For this review, take the finished solid that the model builds, in its own axes (mm). A direction names the side the tool comes from. Round coordinates to 2 decimals unless told otherwise and drop trailing zeros. Order: outer loops, then holes, each group sorted by start corner. A loop starts at its lowest first (then second) coordinate and runs counter-clockwise, first axis right, second up.
```python
from build123d import *

# Parameters (mm, degrees)
ESQUISSE1_W             = 50
ESQUISSE1_H             = 25
BOSS_EXTRU_1_DEPTH      = 12.5
ESQUISSE2_R             = 5
BOSS_EXTRU_2_DEPTH      = 10
BOSS_EXTRU_2_TAPER      = 10
ESQUISSE4_R             = 5
BOSS_EXTRU_3_DEPTH      = 10
BOSS_EXTRU_3_TAPER      = 10
ENL_V_MAT_EXTRU_5_DEPTH = 26
ESQUISSE14_R            = 1.5
ENL_V_MAT_EXTRU_6_DEPTH = 4
ENL_V_MAT_EXTRU_6_TAPER = 10


with BuildPart() as part:
    # Esquisse1 → Boss.-Extru.1 (new body)
    with BuildSketch(Plane(origin=(0, 0, 0), x_dir=(1, 0, 0), z_dir=(0, 1, 0))):
        Rectangle(ESQUISSE1_W, ESQUISSE1_H)
    extrude(amount=-BOSS_EXTRU_1_DEPTH)

    # Esquisse2 → Boss.-Extru.2 (add)
    with BuildSketch(Plane.XZ.offset(12.5)):
        with Locations((17, 4.5)):
            Circle(ESQUISSE2_R)
    extrude(amount=BOSS_EXTRU_2_DEPTH, taper=BOSS_EXTRU_2_TAPER)

    # Esquisse4 → Boss.-Extru.3 (add)
    with BuildSketch(Plane.XZ.offset(12.5)):
        with Locations((-17, -4.5)):
            Circle(ESQUISSE4_R)
    extrude(amount=BOSS_EXTRU_3_DEPTH, taper=BOSS_EXTRU_3_TAPER)

    # Esquisse6 → Enlèvement de matière-Révolution1 (revolve, cut)
    with BuildSketch(Plane.XY):
        with BuildLine():
            Line((0, -20), (0, -5))
            ThreePointArc((0, -5), (-7.5, -12.5), (0, -20))
        make_face()
    revolve(axis=Axis((0, -20, 0), (0, 1, 0)), mode=Mode.SUBTRACT)

    # Esquisse8 → Enlèvement de matière-Révolution2 (revolve, cut)
    with BuildSketch(Plane.XY):
        with BuildLine():
            Line((8, -12.5), (10, -12.5))
            ThreePointArc((10, -12.5), (9, -11.5), (8, -12.5))
        make_face()
    revolve(axis=Axis((0, -20, 0), (0, 1, 0)), mode=Mode.SUBTRACT)

    # Esquisse13 → Enlèv. mat.-Extru.5 (cut, through all)
    with BuildSketch(Plane(origin=(0, 0, -12.5), x_dir=(-1, 0, 0), z_dir=(0, 0, -1))):
        Polygon((20, 0), (20, -7.5), (10, -7.5), (10, -2.5), (-10, -2.5), (-10, -7.5), (-20, -7.5), (-20, 0), align=None)
    extrude(amount=-ENL_V_MAT_EXTRU_5_DEPTH, mode=Mode.SUBTRACT)

    # Esquisse14 → Enlèv. mat.-Extru.6 (cut)
    with BuildSketch(Plane.XY.offset(12.5)):
        with Locations((0, -12.5)):
            Circle(ESQUISSE14_R)
    extrude(amount=-ENL_V_MAT_EXTRU_6_DEPTH, taper=ENL_V_MAT_EXTRU_6_TAPER, mode=Mode.SUBTRACT)


solid = part.part
```
Q1. Take a section at B-B, the plane y = -10.25. State the section outline as (x, z) points, plus the area to 3 significant figures.
Q2. Clearance check with a flat-ended pin moving along its axis: pin 1 (6 mm diameter, centred on x = -2.5, z = 3.5, fed in from +Y). State where the tip first meets the part, or that it passes through.
Q3. Tool access review of faces 1 (the face through (5, -12.5, 6)), 2 (the face through (0, -2.5, 0)), 3 (the face through (-6, -12.5, -9)), 4 (the face through (22, 0, 0)): name each direction out of +Z, -Z, +X, -X, +Y, -Y from which nothing blocks a thin tool from reaching the whole face with its end or side.
Q4. Wall thickness on line 1 (X direction, y = -3.5, z = -5); line 2 (X direction, y = -1.5, z = 0.5); line 3 (Y direction, x = -18.5, z = -10.25): over which ranges is each line inside the solid? List them lowest first.
Q5. Take a section at C-C, the plane x = 0. State the section outline as (y, z) points, plus the area to 3 significant figures.
Q6. Take a section at A-A, the plane x = -17. State the section outline as (y, z) points.
Working result:
1. outline: (-25, -12.5) - (25, -12.5) - (25, 12.5) - (-25, 12.5) - close; hole circle Ø14.31 at (0, 0)
1. area: 1,090 mm2
2. pin 1: stops at y = -2.5
3. face 1: +Z, -Z, -Y
3. face 2: +Z, -Z, +Y
3. face 3: -Y
3. face 4: +Z, -Z, +X, -X, +Y
4. line 1: x = -25 to -20, -10 to 10, 20 to 25
4. line 2: x = -25 to -20, 20 to 25
4. line 3: y = -12.5 to -7.5
5. outline: (-12.5, -12.5) - (-2.5, -12.5) - (-2.5, 12.5) - (-11, 12.5) - (-11.56, 9.34) arc R1 cw to (-12.5, 8) - (-12.5, 7.5) arc R7.5 cw to (-12.5, -7.5) - (-12.5, -8) arc R1 cw to (-12.5, -10) - close
5. area: 155 mm2
6. outline: (-22.5, -7.74) - (-12.5, -9.5) - (-12.5, -12.5) - (-7.5, -12.5) - (-7.5, 12.5) - (-12.5, 12.5) - (-12.5, 0.5) - (-22.5, -1.26) - close
